from build123d import *

# Parameters (mm, degrees)
F0_W     = 220
F0_H     = 510
F1_DEPTH = 22
F2_SIZE  = 21.99999


# Not quite as in the source:
# - a fillet or chamfer is up to 0.001 mm smaller than in the source, because OpenCascade refuses the exact size


with BuildPart() as f1:
    # F0 (on Right) → F1 (new body)
    with BuildSketch(Plane.YZ):
        Rectangle(F0_W, F0_H)
    extrude(amount=F1_DEPTH)

    # F2 (size 22 in the source; OpenCascade refuses exactly that, so slightly less here)
    f2_edges = [f1.edges().sort_by_distance(p)[0] for p in [
        (0, 0, 255),
        (0, 110, 0),
        (0, 0, -255),
        (0, -110, 0),
    ]]
    chamfer(f2_edges, length=F2_SIZE)


solid = f1.part
Verification items for the finished model (mm, model axes). Coordinates: 2 decimals unless noted, no trailing zeros. Loops run counter-clockwise (first coordinate to the right, second up) from the corner with the lowest first, then second, coordinate; pieces in that order, holes last. Notation, with made-up numbers: (13.25, -12) -> (55.25, -12) arc R31 cw to (55.25, 13) -> close; hole circle Ø8 at (47.25, -18.5). An arc over 180 degrees is marked (long way). Answer as a JSON object with one key per item and string values. Group by question number.
Item 1: Mould release check, pull along X, two halves, no side actions. Record for faces 1 (the flat face through (22, -2, 4)), 2 (the flat face through (11, -2, -244)): +X half, -X half, draft (parallel to the pull), parting line (faces both ways), or undercut.
Item 2: Scan lines: probe 1 along Y at (x, z) = (5.5, 23); probe 2 along Z at (x, y) = (16.75, 82); probe 3 along Y at (x, z) = (6.5, 162). Record each from-to range of solid material in increasing order.
Item 3: Sectioned sample at C-C on x = 13.25. Record the boundary of the cut face in (y, z), plus the area to 3 significant figures.
Item 4: Depth check by flat-ended pin: pin 1 (5 mm diameter, centred on x = 4, y = 22.5, fed in from +Z); pin 2 (4 mm diameter, centred on x = 8, y = -71.5, fed in from -Z); pin 3 (1.5 mm diameter, centred on x = 14, z = -72.5, fed in from -Y). Enter the tip coordinate at first touch or a pass-through.
Evaluation:
{
 "1": {"face 1": "+X half", "face 2": "-X half"},
 "2": {"probe 1": "y = -93.5 to 93.5", "probe 2": "z = -249.75 to 249.75", "probe 3": "y = -94.5 to 94.5"},
 "3": {"outline": "(-101.25, -246.25) -> (101.25, -246.25) -> (101.25, 246.25) -> (-101.25, 246.25) -> close", "area": "99,700 mm²"},
 "4": {"pin 1": "stops at z = 239.5", "pin 2": "stops at z = -243", "pin 3": "stops at y = -102.75"}
}
